```python
from build123d import *

# Parameters (mm, degrees)
SKETCH1_R           = 20
BOSS_EXTRUDE1_DEPTH = 3
FILLET1_R           = 15


with BuildPart() as part:
    # Sketch1 → Boss-Extrude1 (new body)
    with BuildSketch(Plane(origin=(0, 0, 0), x_dir=(1, 0, 0), z_dir=(0, 1, 0))):
        Polygon((-286.26, 15), (-410.653398282, 10.606601718), (-421.26, 0), (-410.653398282, -10.606601718), (-286.26, -15), (-281.866601718, -139.393398282), (-271.26, -150), (-260.653398282, -139.393398282), (-256.26, -15), (-131.866601718, -10.606601718), (-121.26, 0), (-131.866601718, 10.606601718), (-256.26, 15), (-260.653398282, 139.393398282), (-271.26, 150), (-281.866601718, 139.393398282), align=None)
        with Locations(Location((-271.26, 0, 0), (0, 0, 270))):
            Circle(SKETCH1_R, mode=Mode.SUBTRACT)
    extrude(amount=BOSS_EXTRUDE1_DEPTH)

    # Fillet1
    fillet1_edges = [part.edges().sort_by_distance(p)[0] for p in [
        (-256.26, 1.5, -15),
        (-256.26, 1.5, 15),
        (-286.26, 1.5, 15),
        (-286.26, 1.5, -15),
    ]]
    fillet(fillet1_edges, radius=FILLET1_R)


solid = part.part
```
Can you work these out from the model? Positions are in its coordinate system, mm. Round coordinates to 2 decimals unless told otherwise and drop trailing zeros. Loops run counter-clockwise (first coordinate to the right, second up) from the corner with the lowest first, then second, coordinate; pieces in that order, holes last. Notation, with made-up numbers: M 89,88.5 L 115,88.5 A17 ccw 115,101.5 Z; hole C -38.75,28 d6. An arc over 180 degrees is marked long. Answer in a Markdown table with one row per item.
1. If we section it at A-A, the plane y = 1.15: Please give me the cut outline in (x, z).
Established:
| item | result |
|---|---|
| outline | M -421.26,0 L -410.65,-10.61 L -300.23,-14.51 A15 cw -285.77,-28.97 L -281.87,-139.39 L -271.26,-150 L -260.65,-139.39 L -256.75,-28.97 A15 cw -242.29,-14.51 L -131.87,-10.61 L -121.26,0 L -131.87,10.61 L -242.29,14.51 A15 cw -256.75,28.97 L -260.65,139.39 L -271.26,150 L -281.87,139.39 L -285.77,28.97 A15 cw -300.23,14.51 L -410.65,10.61 Z; hole C -271.26,0 d40 |
2. I'm going to push flat-ended pins straight in: pin 1 Ø24 at (x, z) = (-271.26, 0) entering from +Y; pin 2 Ø1.5 at (x, y) = (-389.5, 2) entering from +Z. Where does each tip first touch, or does it pass through?
Established:
| item | result |
|---|---|
| pin 1 | through |
| pin 2 | z = 11.38 |
3. Thinking about a two-plate mould opening in Z: for faces 1 (the face through (-290.26, 1.52, -18.78)), 2 (the face through (-126.64, 1.48, 5.38)), 3 (the face through (-290.784, 1.479, -4.336)), which applies, pulls with the +Z half, pulls with the -Z half, needs draft (parallel to the pull), parting line crosses it, or undercut?
Established:
| item | result |
|---|---|
| face 1 | pulls with the -Z half |
| face 2 | pulls with the +Z half |
| face 3 | undercut |
4. If we section it at D-D, the plane z = 40.5: Please give me the cut outline in (x, y).
Established:
| item | result |
|---|---|
| outline | M -285.36,0 L -257.16,0 L -257.16,3 L -285.36,3 Z |
5. If we section it at C-C, the plane x = -276: Please give me the cut outline in (y, z), plus the area to 3 significant figures.
Established:
| item | result |
|---|---|
| outline | M 0,-145.26 L 3,-145.26 L 3,-19.43 L 0,-19.43 Z; M 0,19.43 L 3,19.43 L 3,145.26 L 0,145.26 Z |
| area | 755 mm² |
6. Please list where these lines run through material, in increasing order: line 1 (X direction, y = 0.7, z = 0); line 2 (Z direction, x = -331, y = 2.3); line 3 (X direction, y = 1.3, z = -54). Write a range as from..to.
Established:
| item | result |
|---|---|
| line 1 | -421.26..-291.26, -251.26..-121.26 |
| line 2 | -13.42..13.42 |
| line 3 | -284.88..-257.64 |
7. If we section it at B-B, the plane z = -5: Please give me the cut outline in (x, y), plus the area to 3 significant figures.
Established:
| item | result |
|---|---|
| outline | M -416.26,0 L -290.62,0 L -290.62,3 L -416.26,3 Z; M -251.9,0 L -126.26,0 L -126.26,3 L -251.9,3 Z |
| area | 754 mm² |
